Autodesk Inventor part; units mm, degrees
ref_plane "Plano inicial" through (0, 0, 0) normal (1, 0, 0) x (0, 1, 0)
ref_plane "XZ Plane" through (0, 0, 0) normal (0, 1, 0) x (-1, 0, 0)
ref_plane "XY Plane" through (0, 0, 0) normal (0, 0, 1) x (1, 0, 0)
sketch "Boceto principal" plane through (0, 0, 0) normal (0, 0, 1) x (1, 0, 0)
  line L0 (0, 0) -> (440.47, 0)
  line L1 (11.5, 5.5) -> (11.5, 6.5)
  line L2 (11.5, 6.5) -> (48.5, 6.5)
  line L3 (0, 5.5) -> (11.5, 5.5)
  line L4 (186.707, 7.5) -> (186.707, 6.5)
  line L5 (48.5, 7.5) -> (186.707, 7.5)
  line L6 (0, 0) -> (0, 5.5)
  line L7 (48.5, 6.5) -> (48.5, 7.5)
  line L8 (186.707, 6.5) -> (207, 6.5)
  line L9 (207, 6.5) -> (287.1, 6.5)
  line L10 (287.1, 6.5) -> (391.97, 6.5)
  line L11 (428.97, 6.5) -> (428.97, 5.5)
  line L12 (391.97, 6.5) -> (428.97, 6.5)
  line L13 (440.47, 5.5) -> (440.47, 0)
  line L14 (428.97, 5.5) -> (440.47, 5.5)
  dimension "d3" = 13
  dimension "d4" = 11
  dimension "d5" = 15
  dimension "d10" = 13
  dimension "d11" = 13
  dimension "d12" = 13
  dimension "d13" = 13
  dimension "d41" = 11
revolve "Revolución1" add sketch "Boceto principal" angle 360 about axis through (0, 0, 0) along (1, 0, 0)
fillet "Fillet7" radius 0.5 1 edges at (428.97, -5.5, 0)
chamfer "Chamfer9" distance 0.5 angle 45 1 edges at (440.47, -5.5, 0) measured on face at (433.1367, 5.4288, -0.8823)
chamfer "Chamfer2" distance 0.5 angle 45 1 edges at (0, -5.5, 0) measured on face at (3.8333, 5.4288, -0.8823)
fillet "Fillet1" radius 0.5 1 edges at (11.5, -5.5, 0)
fillet "Fillet2" radius 0.5 1 edges at (48.5, -6.5, 0)
chamfer "Chamfer3" distance 0.5 angle 45 1 edges at (48.5, -7.5, 0) measured on face at (94.569, 7.4029, -1.2031)
chamfer "Chamfer4" distance 0.5 angle 45 1 edges at (186.707, -7.5, 0) measured on face at (94.9023, 7.4757, -0.6035)
fillet "Fillet3" radius 0.5 1 edges at (186.707, -6.5, 0)
chamfer "Chamfer8" distance 0.5 angle 45 1 edges at (428.97, -6.5, 0) measured on face at (404.3033, 6.4158, -1.0427)
chamfer "Chaflán1" distance 0.5 angle 45 1 edges at (11.5, -6.5, 0) measured on face at (23.6667, 6.4789, -0.523)
properties part number "Eje" material "Steel"
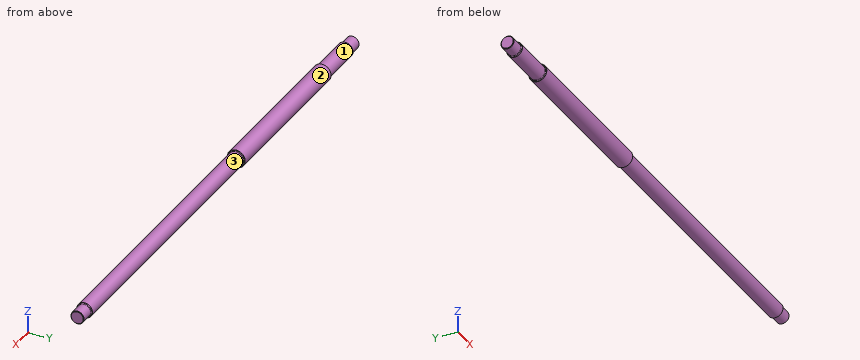
Here's how the part is built. I have some questions about the finished solid (model axes, mm). Face numbers are marked on the shaded views. A direction names the side the tool comes from. Coordinates: 2 decimals unless noted, no trailing zeros. Loops run counter-clockwise (first coordinate to the right, second up) from the corner with the lowest first, then second, coordinate; pieces in that order, holes last. Notation, with made-up numbers: (46.5, 74) - (81.5, 74) arc R22 cw to (81.5, 80) - close; hole circle Ø1 at (70.5, 70). An arc over 180 degrees is marked (long way). Answer as CSV lines item,"result".
Q1. If I drill on L1, parallel to X at y = -2, z = 5.5; L2, parallel to Y at x = 212, z = -0.5; L3, parallel to Z at x = 376, y = -4.5, over which ranges is the centre line in solid material (lowest first)? Write a range as [from, to].
Response:
L1,"[11.48, 428.99]"
L2,"[-6.48, 6.48]"
L3,"[-4.69, 4.69]"
Q2. If we section it at A-A, the plane x = 250: Write out the boundary of the cut face in (y, z).
Response:
outline,"circle Ø13 at (0, 0)"
Q3. For pin 1 (1.5 mm diameter, centred on x = 385.5, z = 4, fed in from -Y); pin 2 (1 mm diameter, centred on y = -4.5, z = -4.5, fed in from -X); pin 3 (3 mm diameter, centred on x = 175, y = 6, fed in from -Z), each with a flat end and sliding along its axis, tell me the tip position at first contact or that it passes through.
Response:
pin 1,"y = -5.63"
pin 2,"x = 11.48"
pin 3,"z = -6"
Q4. For the marked faces 1, 2 and 3, which set-ups out of +Z, -Z, +X, -X, +Y, -Y let a thin tool reach every point of the face, with its end or its side?
Response:
face 1,"-X"
face 2,"+X, -X"
face 3,"+X"
